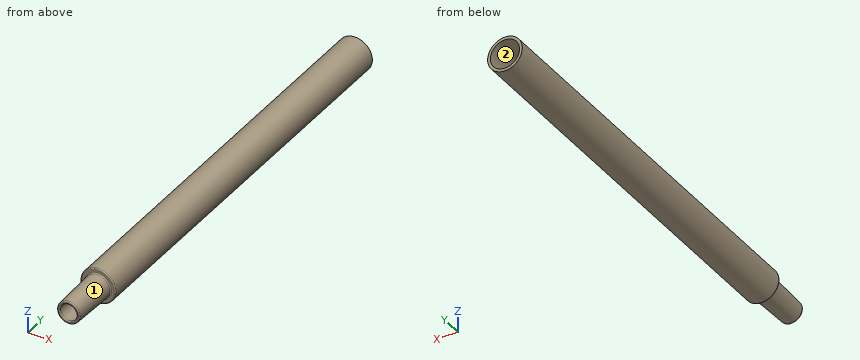
from build123d import *

# Parameters (mm, degrees)
VERRUNDUNG1_R = 0.2


with BuildPart() as part:
    # Skizze1 → Rotation1 (revolve)
    with BuildSketch(Plane.XY):
        Polygon((-2.6, 82.5), (-3.1, 82.5), (-3.1, 8.5), (-2.25, 8.5), (-2, 0), (-1.5, 0), (-1.764705882, 9), (-2.6, 9), align=None)
    revolve(axis=Axis((0, 0, 0), (0, -1, 0)))

    # Verrundung1
    verrundung1_edges = [part.edges().sort_by_distance(p)[0] for p in [
        (1.5, 0, 0),
        (2, 0, 0),
        (2.25, 8.5, 0),
        (3.1, 8.5, 0),
    ]]
    fillet(verrundung1_edges, radius=VERRUNDUNG1_R)


solid = part.part
Input: part model. Units: mm. Frame: model coordinates. Face numbers are marked on the shaded views. Give positions to 0.01 mm unless a question says otherwise; leave off trailing zeros. Order: outer loops, then holes, each group sorted by start corner. A loop starts at its lowest first (then second) coordinate and runs counter-clockwise, first axis right, second up. Notation, with made-up numbers: (40, 22.5) - (58, 22.5) arc R20 ccw to (58, 28.5) - close; hole circle Ø6 at (-29, 59.25). An arc over 180 degrees is marked (long way). Write each question's results on one line, items separated by ' | '.
Item 1: Section A-A (x = 0). Return loops of the section in (y, z).
A:
outline: (0, -1.81) arc R0.2 ccw to (0.19, -2.01) - (8.31, -2.24) arc R0.2 cw to (8.5, -2.44) - (8.5, -2.9) arc R0.2 ccw to (8.7, -3.1) - (82.5, -3.1) - (82.5, -2.6) - (9, -2.6) - (9, -1.76) - (0.21, -1.51) arc R0.2 ccw to (0, -1.71) - close; (0, 1.71) arc R0.2 ccw to (0.21, 1.51) - (9, 1.76) - (9, 2.6) - (82.5, 2.6) - (82.5, 3.1) - (8.7, 3.1) arc R0.2 ccw to (8.5, 2.9) - (8.5, 2.44) arc R0.2 cw to (8.31, 2.24) - (0.19, 2.01) arc R0.2 ccw to (0, 1.81) - close
Item 2: Section C-C (y = 15.5). Return loops of the section in (x, z), and give its area (3 significant figures).
A:
outline: circle Ø6.2 at (0, 0); hole circle Ø5.2 at (0, 0) | area: 8.95 mm^2
Item 3: Contact query for flat-ended pins moving along their axis: pin 1 Ø3 at (x, z) = (1.5, -2) entering from -Y; pin 2 Ø1 at (x, y) = (1, 10.5) entering from -Z. Output: stop coordinate, or through.
A:
pin 1: stops at y = 0 | pin 2: stops at z = -3.06
Item 4: Material intervals for line 1 along Z through (x, y) = (0, 64); line 2 along X through (y, z) = (41.5, -1.5), sorted ascending.
A:
line 1: z = -3.1 to -2.6, 2.6 to 3.1 | line 2: x = -2.71 to -2.12, 2.12 to 2.71
Item 5: Section B-B (z = 0). Return loops of the section in (x, y), and give its area (3 significant figures).
A:
outline: (-3.1, 8.7) arc R0.2 ccw to (-2.9, 8.5) - (-2.44, 8.5) arc R0.2 cw to (-2.24, 8.31) - (-2.01, 0.19) arc R0.2 ccw to (-1.81, 0) - (-1.71, 0) arc R0.2 ccw to (-1.51, 0.21) - (-1.76, 9) - (-2.6, 9) - (-2.6, 82.5) - (-3.1, 82.5) - close; (1.51, 0.21) arc R0.2 ccw to (1.71, 0) - (1.81, 0) arc R0.2 ccw to (2.01, 0.19) - (2.24, 8.31) arc R0.2 cw to (2.44, 8.5) - (2.9, 8.5) arc R0.2 ccw to (3.1, 8.7) - (3.1, 82.5) - (2.6, 82.5) - (2.6, 9) - (1.76, 9) - close | area: 83.3 mm^2
Item 6: Draft query along Z for the marked faces 1 and 2. Return one class per face: released by +Z, released by -Z, zero draft, split by the parting line, or undercut.
A:
face 1: split by the parting line | face 2: undercut
